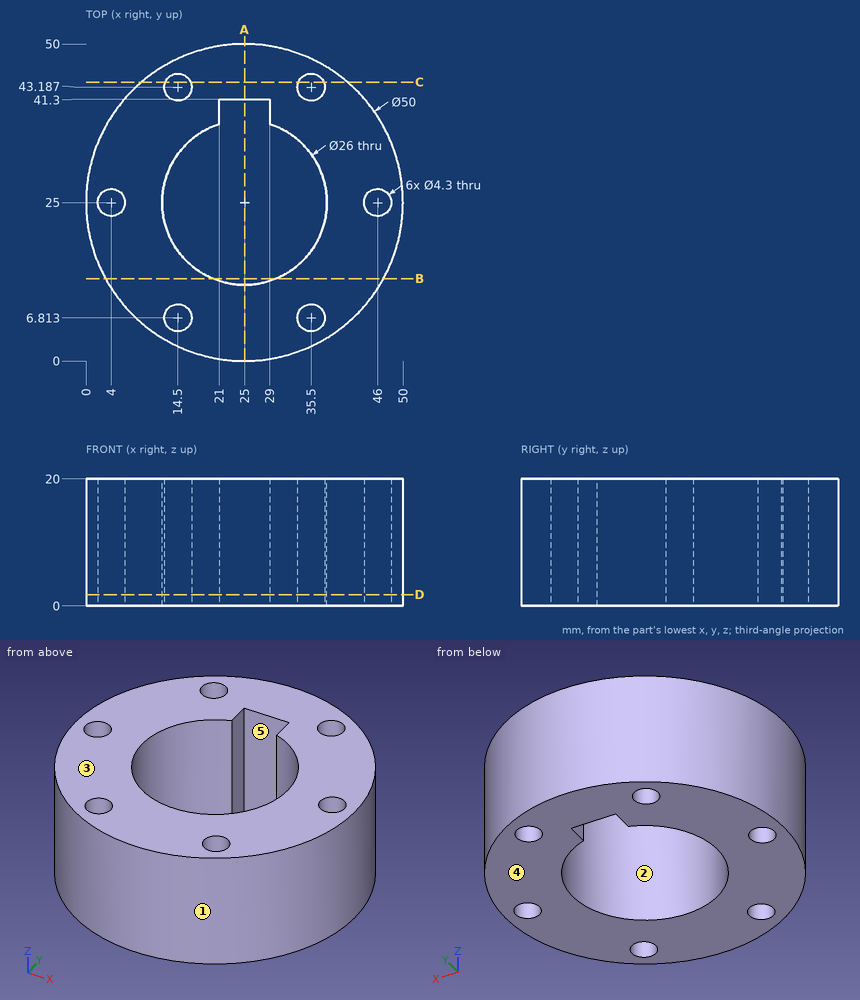
Part print with two shaded views. Sizes in mm from the minimum x, y, z corner. A direction names the side the tool comes from. Round coordinates to 2 decimals unless told otherwise and drop trailing zeros. Order: outer loops, then holes, each group sorted by start corner. A loop starts at its lowest first (then second) coordinate and runs counter-clockwise, first axis right, second up. Notation, with made-up numbers: M -17,-9.5 L 33,-9.5 A8 ccw 33,0.5 Z; hole C -31,14.5 d4. An arc over 180 degrees is marked long. Put each result on its own line as item: value. Start each with the question number.
1. Two-plate mould, pull along X, no slides. Class the marked faces 1, 2 and 3: +X half, -X half, draft (parallel to the pull), parting line (faces both ways), or undercut.
2. Slice it at D-D on z = 1.75. List the corners of the cut face in (x, y).
3. Tool access for the marked faces 4 and 5: list every direction of +Z, -Z, +X, -X, +Y, -Y with a clear straight run to the whole face (end or side of a thin tool).
4. Drop flat-ended pins along their axis: pin 1 (4 mm diameter, centred on y = 18.5, z = 6.5, fed in from +X); pin 2 (2 mm diameter, centred on y = 38.5, z = 8.5, fed in from -X); pin 3 (9 mm diameter, centred on x = 23.5, z = 5.5, fed in from -Y). Give the stop position or say it passes through.
5. Drill centre lines: probe 1 along Y at (x, z) = (14.5, 9.25) (1 decimal); probe 2 along X at (y, z) = (44.5, 13) (1 decimal); probe 3 along Y at (x, z) = (13.5, 18) (1 decimal). Where is each one in solid material? Low to high. Write a range as [from, to].
6. Slice it at A-A on x = 25. List the corners of the cut face in (y, z), then the cut area to 3 significant figures.
7. Slice it at B-B on y = 13. List the corners of the cut face in (x, z), then the cut area to 3 significant figures.
8. Slice it at C-C on y = 44. List the corners of the cut face in (x, z), then the cut area to 3 significant figures.
Findings:
1. face 1: parting line
1. face 2: undercut
1. face 3: draft
2. outline: C 25,25 d50; hole C 4,25 d4.3; hole C 14.5,6.81 d4.3; hole C 14.5,43.19 d4.3; hole M 21,37.37 A13 ccw long 29,37.37 L 29,41.3 L 21,41.3 Z; hole C 35.5,6.81 d4.3; hole C 35.5,43.19 d4.3; hole C 46,25 d4.3
3. face 4: -Z, +X, -X, +Y, -Y
3. face 5: +Z, -Z
4. pin 1: x = 49.59
4. pin 2: x = 3.35
4. pin 3: y = 0
5. probe 1: [2.3, 4.7], [9, 17.3], [32.7, 41], [45.3, 47.7]
5. probe 2: [9.4, 12.8], [16.2, 33.8], [37.2, 40.6]
5. probe 3: [2.8, 4.9], [8.7, 18.9], [31.1, 41.3], [45.1, 47.2]
6. outline: M 0,0 L 12,0 L 12,20 L 0,20 Z; M 41.3,0 L 50,0 L 50,20 L 41.3,20 Z
6. area: 414 mm2
7. outline: M 3.07,0 L 20,0 L 20,20 L 3.07,20 Z; M 30,0 L 46.93,0 L 46.93,20 L 30,20 Z
7. area: 677 mm2
8. outline: M 8.75,0 L 12.51,0 L 12.51,20 L 8.75,20 Z; M 16.49,0 L 33.51,0 L 33.51,20 L 16.49,20 Z; M 37.49,0 L 41.25,0 L 41.25,20 L 37.49,20 Z
8. area: 491 mm2
